Work out the finished part from the listing and answer in its coordinate system (mm). Face numbers are marked on the shaded views. A direction names the side the tool comes from. Give positions to 0.01 mm unless a question says otherwise; leave off trailing zeros. Loops run counter-clockwise (first coordinate to the right, second up) from the corner with the lowest first, then second, coordinate; pieces in that order, holes last. Notation, with made-up numbers: (-19, 69.25) -> (10, 69.25) arc R18 ccw to (10, 83.25) -> close; hole circle Ø6 at (39, 68). An arc over 180 degrees is marked (long way). Answer as CSV lines item,"result". Start each with the question number.
1. A tool of negligible diameter and unlimited length cuts with its end or side. For the marked faces 1 and 2, from which of +Z, -Z, +X, -X, +Y, -Y can it reach the whole face along a straight path? Write none if from no direction.
2. Find section B-B, the plane z = 23. Give the vertices of the cut face in (x, y) (3 decimals).
3. Find the intervals of material crossed by line 1 along Z through (x, y) = (-6.5, -66); line 2 along Y through (x, z) = (4.25, 35.5); line 3 along Z through (x, y) = (-3, -40.5), in increasing order.
4. Find section D-D, the plane y = -64.5. Give the vertices of the cut face in (x, z), and give its area (3 significant figures).
5. Determine the mould class of the marked faces 3, 4 and 5 for opening direction X: +X half, -X half, draft (parallel to the pull), parting line (faces both ways), or undercut.
6. Find section C-C, the plane y = -46.5. Give the vertices of the cut face in (x, z) (3 decimals), and give its area (3 significant figures).
7. Flat-ended cylindrical pins translate along their axes: pin 1 Ø1.5 at (x, y) = (1, -28.5) entering from +Z; pin 2 Ø15 at (x, z) = (0.02, -1.33) entering from +Y. Find the tip coordinate at first contact, or state that the pin passes through.
8. Find section A-A, the plane x = -4.75. Give the vertices of the cut face in (y, z) (3 decimals), and give its area (3 significant figures).
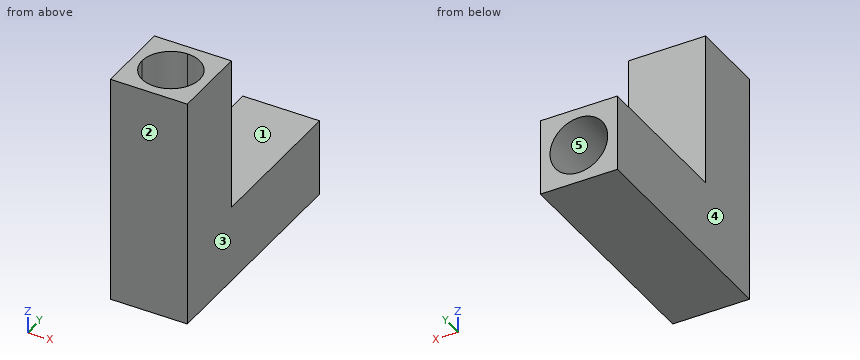
from build123d import *

# Parameters (mm, degrees)
F0_W     = 25.4
F0_H     = 25.4
F1_DEPTH = 76.2
F2_W     = 25.4
F2_H     = 25.4
F3_DEPTH = 50.8
F5_DEPTH = 69.85
F7_R     = 9.525
F8_DEPTH = 69.85


with BuildPart() as f1:
    # F0 (on Front) → F1 (new body)
    with BuildSketch(Plane.XZ):
        with Locations((0.0199213878, -1.3326740591)):
            Rectangle(F0_W, F0_H)
    extrude(amount=F1_DEPTH)

    # F2 (on face) → F3 (join)
    with BuildSketch(Plane.XY.offset(11.3673259409)):
        with Locations((0.0199213878, -63.5)):
            Rectangle(F2_W, F2_H)
    extrude(amount=F3_DEPTH)

    # F4 (on face) → F5 (cut)
    with BuildSketch(Plane(origin=(0, 0, 0), x_dir=(-1, 0, 0), z_dir=(0, 1, 0))):
        with BuildLine():
            ThreePointArc((-0.0199213878, -10.8576740591), (6.715270703, -8.0678661499), (9.5050786122, -1.3326740591))
            Line((9.5050786122, -1.3326740591), (-0.0199213878, -1.3326740591))
            Line((-0.0199213878, -1.3326740591), (-0.0199213878, -10.8576740591))
        make_face()
        with BuildLine():
            Line((-0.0199213878, -10.8576740591), (-0.0199213878, -1.3326740591))
            Line((-0.0199213878, -1.3326740591), (-9.5449213878, -1.3326740591))
            ThreePointArc((-9.5449213878, -1.3326740591), (-6.7551134786, -8.0678661499), (-0.0199213878, -10.8576740591))
        make_face()
        with BuildLine():
            Line((-0.0199213878, -1.3326740591), (9.5050786122, -1.3326740591))
            ThreePointArc((9.5050786122, -1.3326740591), (-0.0199213878, 8.1923259409), (-9.5449213878, -1.3326740591))
            Line((-9.5449213878, -1.3326740591), (-0.0199213878, -1.3326740591))
        make_face()
    extrude(amount=-F5_DEPTH, mode=Mode.SUBTRACT)

    # F7
    f7_edges = [f1.edges().sort_by_distance(p)[0] for p in [
        (9.544921, -69.85, -1.332674),
    ]]
    fillet(f7_edges, radius=F7_R)

    # F6 (on face) → F8 (cut)
    with BuildSketch(Plane.XY.offset(62.1673259409)):
        with BuildLine():
            ThreePointArc((9.5449213878, -63.5), (6.7551134786, -56.7648079092), (0.0199213878, -53.975))
            Line((0.0199213878, -53.975), (0.0199213878, -63.5))
            Line((0.0199213878, -63.5), (0.0199213878, -73.025))
            ThreePointArc((0.0199213878, -73.025), (6.7551134786, -70.2351920908), (9.5449213878, -63.5))
        make_face()
        with BuildLine():
            Line((0.0199213878, -73.025), (0.0199213878, -63.5))
            Line((0.0199213878, -63.5), (-9.5050786122, -63.5))
            ThreePointArc((-9.5050786122, -63.5), (-6.715270703, -70.2351920908), (0.0199213878, -73.025))
        make_face()
        with BuildLine():
            Line((0.0199213878, -63.5), (0.0199213878, -53.975))
            ThreePointArc((0.0199213878, -53.975), (-6.715270703, -56.7648079092), (-9.5050786122, -63.5))
            Line((-9.5050786122, -63.5), (0.0199213878, -63.5))
        make_face()
    extrude(amount=-F8_DEPTH, mode=Mode.SUBTRACT)


solid = f1.part
Resolved:
1,face 1,"+Z, +X, -X, +Y"
1,face 2,"+Z, -Z, +X, -X, -Y"
2,outline,"(-12.68, -76.2) -> (12.72, -76.2) -> (12.72, -50.8) -> (-12.68, -50.8) -> close; hole circle Ø19.05 at (0.02, -63.5)"
3,line 1,"z = -14.03 to -7.68"
3,line 2,"y = -76.2 to -72.03, -54.97 to -50.8"
3,line 3,"z = -14.03 to -10.37, 7.7 to 11.37"
4,outline,"(-12.68, -14.03) -> (12.72, -14.03) -> (12.72, 62.17) -> (9.49, 62.17) -> (9.49, -7.68) -> (5.76, -7.68) arc R8.56 cw to (-5.72, -7.68) -> (-9.45, -7.68) -> (-9.45, 62.17) -> (-12.68, 62.17) -> close"
4,area,"595 mm^2"
5,face 3,"+X half"
5,face 4,"-X half"
5,face 5,"undercut"
6,outline,"(-12.68, -14.033) -> (12.72, -14.033) -> (12.72, 11.367) -> (-12.68, 11.367) -> close; hole circle Ø19.05 at (0.02, -1.333)"
6,area,"360 mm^2"
7,pin 1,"stops at z = 11.37"
7,pin 2,"stops at y = -66.2"
8,outline,"(-76.2, -14.033) -> (0, -14.033) -> (0, -9.577) -> (-60.325, -9.577) arc R8.245 cw to (-65.583, -7.683) -> (-71.745, -7.683) -> (-71.745, 62.167) -> (-76.2, 62.167) -> close; (-55.255, 6.912) -> (0, 6.912) -> (0, 11.367) -> (-50.8, 11.367) -> (-50.8, 62.167) -> (-55.255, 62.167) -> close"
8,area,"1,150 mm^2"
